```python
from build123d import *

# Parameters (mm, degrees)
F0_W     = 6
F0_H     = 20
F1_DEPTH = 9
F2_DEPTH = 6


with BuildPart() as f1:
    # F0 (on Front) → F1 (new body)
    with BuildSketch(Plane.XZ):
        Polygon((-37.5, -22), (-37.5, -30), (-29.5, -30), (-29.5, -26.6002), (-30.857, -26.6002), (-30.857, -25), (-29.5, -25), (-29.5, -23.65), (-27.214, -23.65), (-27.214, -25), (-25.857, -25), (-25.857, -26.6002), (-27.214, -26.6002), (-27.214, -30), (27.214, -30), (27.214, -26.6002), (25.857, -26.6002), (25.857, -25), (27.214, -25), (27.214, -23.65), (29.5, -23.65), (29.5, -25), (30.857, -25), (30.857, -26.6002), (29.5, -26.6002), (29.5, -30), (37.5, -30), (37.5, -22), (34.1002, -22), (34.1002, -23.357), (32.5, -23.357), (32.5, -22), (31.15, -22), (31.15, -19.714), (32.5, -19.714), (32.5, -18.357), (34.1002, -18.357), (34.1002, -19.714), (37.5, -19.714), (37.5, -10), (37.5, 10), (37.5, 19.714), (34.1002, 19.714), (34.1002, 18.357), (32.5, 18.357), (32.5, 19.714), (31.15, 19.714), (31.15, 22), (32.5, 22), (32.5, 23.357), (34.1002, 23.357), (34.1002, 22), (37.5, 22), (37.5, 30), (29.5, 30), (29.5, 26.6002), (30.857, 26.6002), (30.857, 25), (29.5, 25), (29.5, 23.65), (27.214, 23.65), (27.214, 25), (25.857, 25), (25.857, 26.6002), (27.214, 26.6002), (27.214, 30), (-27.214, 30), (-27.214, 26.6002), (-25.857, 26.6002), (-25.857, 25), (-27.214, 25), (-27.214, 23.65), (-29.5, 23.65), (-29.5, 25), (-30.857, 25), (-30.857, 26.6002), (-29.5, 26.6002), (-29.5, 30), (-37.5, 30), (-37.5, 22), (-34.1002, 22), (-34.1002, 23.357), (-32.5, 23.357), (-32.5, 22), (-31.15, 22), (-31.15, 19.714), (-32.5, 19.714), (-32.5, 18.357), (-34.1002, 18.357), (-34.1002, 19.714), (-37.5, 19.714), (-37.5, 10), (-37.5, -10), (-37.5, -19.714), (-34.1002, -19.714), (-34.1002, -18.357), (-32.5, -18.357), (-32.5, -19.714), (-31.15, -19.714), (-31.15, -22), (-32.5, -22), (-32.5, -23.357), (-34.1002, -23.357), (-34.1002, -22), align=None)
        Polygon((-29.5, -26.6002), (-29.5, -30), (-27.214, -30), (-27.214, -26.6002), (-25.857, -26.6002), (-25.857, -25), (-27.214, -25), (-27.214, -23.65), (-29.5, -23.65), (-29.5, -25), (-30.857, -25), (-30.857, -26.6002), align=None)
        Polygon((-37.5, -19.714), (-37.5, -22), (-34.1002, -22), (-34.1002, -23.357), (-32.5, -23.357), (-32.5, -22), (-31.15, -22), (-31.15, -19.714), (-32.5, -19.714), (-32.5, -18.357), (-34.1002, -18.357), (-34.1002, -19.714), align=None)
        Polygon((27.214, -26.6002), (27.214, -30), (29.5, -30), (29.5, -26.6002), (30.857, -26.6002), (30.857, -25), (29.5, -25), (29.5, -23.65), (27.214, -23.65), (27.214, -25), (25.857, -25), (25.857, -26.6002), align=None)
        with Locations((-40.5, 0)):
            Rectangle(F0_W, F0_H)
        Polygon((-37.5, 22), (-37.5, 19.714), (-34.1002, 19.714), (-34.1002, 18.357), (-32.5, 18.357), (-32.5, 19.714), (-31.15, 19.714), (-31.15, 22), (-32.5, 22), (-32.5, 23.357), (-34.1002, 23.357), (-34.1002, 22), align=None)
        Polygon((34.1002, -22), (37.5, -22), (37.5, -19.714), (34.1002, -19.714), (34.1002, -18.357), (32.5, -18.357), (32.5, -19.714), (31.15, -19.714), (31.15, -22), (32.5, -22), (32.5, -23.357), (34.1002, -23.357), align=None)
        with Locations((40.5, 0)):
            Rectangle(F0_W, F0_H)
        Polygon((-27.214, 30), (-29.5, 30), (-29.5, 26.6002), (-30.857, 26.6002), (-30.857, 25), (-29.5, 25), (-29.5, 23.65), (-27.214, 23.65), (-27.214, 25), (-25.857, 25), (-25.857, 26.6002), (-27.214, 26.6002), align=None)
        Polygon((34.1002, 19.714), (37.5, 19.714), (37.5, 22), (34.1002, 22), (34.1002, 23.357), (32.5, 23.357), (32.5, 22), (31.15, 22), (31.15, 19.714), (32.5, 19.714), (32.5, 18.357), (34.1002, 18.357), align=None)
        Polygon((29.5, 30), (27.214, 30), (27.214, 26.6002), (25.857, 26.6002), (25.857, 25), (27.214, 25), (27.214, 23.65), (29.5, 23.65), (29.5, 25), (30.857, 25), (30.857, 26.6002), (29.5, 26.6002), align=None)
    extrude(amount=-F1_DEPTH)

    # F0 (on Front) → F2 (cut)
    with BuildSketch(Plane.XZ):
        Polygon((-37.5, 22), (-37.5, 19.714), (-34.1002, 19.714), (-34.1002, 18.357), (-32.5, 18.357), (-32.5, 19.714), (-31.15, 19.714), (-31.15, 22), (-32.5, 22), (-32.5, 23.357), (-34.1002, 23.357), (-34.1002, 22), align=None)
        Polygon((-27.214, 30), (-29.5, 30), (-29.5, 26.6002), (-30.857, 26.6002), (-30.857, 25), (-29.5, 25), (-29.5, 23.65), (-27.214, 23.65), (-27.214, 25), (-25.857, 25), (-25.857, 26.6002), (-27.214, 26.6002), align=None)
        Polygon((-37.5, -19.714), (-37.5, -22), (-34.1002, -22), (-34.1002, -23.357), (-32.5, -23.357), (-32.5, -22), (-31.15, -22), (-31.15, -19.714), (-32.5, -19.714), (-32.5, -18.357), (-34.1002, -18.357), (-34.1002, -19.714), align=None)
        Polygon((-29.5, -26.6002), (-29.5, -30), (-27.214, -30), (-27.214, -26.6002), (-25.857, -26.6002), (-25.857, -25), (-27.214, -25), (-27.214, -23.65), (-29.5, -23.65), (-29.5, -25), (-30.857, -25), (-30.857, -26.6002), align=None)
        Polygon((27.214, -26.6002), (27.214, -30), (29.5, -30), (29.5, -26.6002), (30.857, -26.6002), (30.857, -25), (29.5, -25), (29.5, -23.65), (27.214, -23.65), (27.214, -25), (25.857, -25), (25.857, -26.6002), align=None)
        Polygon((34.1002, -22), (37.5, -22), (37.5, -19.714), (34.1002, -19.714), (34.1002, -18.357), (32.5, -18.357), (32.5, -19.714), (31.15, -19.714), (31.15, -22), (32.5, -22), (32.5, -23.357), (34.1002, -23.357), align=None)
        Polygon((34.1002, 19.714), (37.5, 19.714), (37.5, 22), (34.1002, 22), (34.1002, 23.357), (32.5, 23.357), (32.5, 22), (31.15, 22), (31.15, 19.714), (32.5, 19.714), (32.5, 18.357), (34.1002, 18.357), align=None)
        Polygon((29.5, 30), (27.214, 30), (27.214, 26.6002), (25.857, 26.6002), (25.857, 25), (27.214, 25), (27.214, 23.65), (29.5, 23.65), (29.5, 25), (30.857, 25), (30.857, 26.6002), (29.5, 26.6002), align=None)
    extrude(amount=-F2_DEPTH, mode=Mode.SUBTRACT)


solid = f1.part
```
Here's how the part is built. I have some questions about the finished solid (model axes, mm). A direction names the side the tool comes from. Coordinates: 2 decimals unless noted, no trailing zeros. Loops run counter-clockwise (first coordinate to the right, second up) from the corner with the lowest first, then second, coordinate; pieces in that order, holes last. Notation, with made-up numbers: (24.5, 31.5) - (43.5, 31.5) arc R8 ccw to (43.5, 37.5) - close; hole circle Ø2 at (30.25, 9). An arc over 180 degrees is marked (long way). Answer as CSV lines item,"result".
Q1. If we section it at B-B, the plane z = 14: Write out the boundary of the cut face in (x, y).
Response:
outline,"(-37.5, 0) - (37.5, 0) - (37.5, 9) - (-37.5, 9) - close"
Q2. If we section it at A-A, the plane y = 8: Write out the boundary of the cut face in (x, z), and give its area (3 significant figures).
Response:
outline,"(-43.5, -10) - (-37.5, -10) - (-37.5, -30) - (37.5, -30) - (37.5, -10) - (43.5, -10) - (43.5, 10) - (37.5, 10) - (37.5, 30) - (-37.5, 30) - (-37.5, 10) - (-43.5, 10) - close"
area,"4,740 mm2"
Q3. For faces 4 (the face through (-41, 4, -10)), 5 (the face through (-31.15, 3, 21)), 6 (the face through (31.15, 3, -21)), 7 (the face through (-37.5, 6.4, 20.1)), 8 (the face through (-33, 3, -18.357)), which set-ups out of +Z, -Z, +X, -X, +Y, -Y let a thin tool reach every point of the face, with its end or its side?
Response:
face 4,"-Z, -X, +Y, -Y"
face 5,"-X, -Y"
face 6,"+X, -Y"
face 7,"+Z, -X, +Y, -Y"
face 8,"-Y"
Q4. We'd pull the mould along Z, two halves only. Please class faces 1 (the face through (-37.5, 6.4, -19.9)), 2 (the face through (1, 4, 30)), 3 (the face through (-33, 3, 18.357)): pulls with the +Z half, pulls with the -Z half, needs draft (parallel to the pull), parting line crosses it, or undercut.
Response:
face 1,"needs draft"
face 2,"pulls with the +Z half"
face 3,"undercut"
Q5. For pin 1 (2 mm diameter, centred on y = 1.5, z = 11.5, fed in from -X); pin 2 (0.7 mm diameter, centred on y = 3, z = 21.5, fed in from +X); pin 3 (5 mm diameter, centred on y = 6, z = 18.5, fed in from +X), each with a flat end and sliding along its axis, tell me the tip position at first contact or that it passes through.
Response:
pin 1,"x = -37.5"
pin 2,"x = 31.15"
pin 3,"x = 37.5"
Q6. If I drill on L1, parallel to X at y = 2.5, z = 25.5; L2, parallel to X at y = 4.75, z = 22.5; L3, parallel to Z at x = -34, y = 3, over which ranges is the centre line in solid material (lowest first)? Write a range as [from, to].
Response:
L1,"[-37.5, -30.86], [-25.86, 25.86], [30.86, 37.5]"
L2,"[-37.5, -34.1], [-32.5, 32.5], [34.1, 37.5]"
L3,"[-30, -23.36], [-18.36, 18.36], [23.36, 30]"
